Check sheet for the modelled part. Datum: model origin and axes. Units: mm. Face numbers are marked on the shaded views. Round coordinates to 2 decimals unless told otherwise and drop trailing zeros. Order: outer loops, then holes, each group sorted by start corner. A loop starts at its lowest first (then second) coordinate and runs counter-clockwise, first axis right, second up. Notation, with made-up numbers: (-5.5, 1.25) -> (37.5, 1.25) arc R15 ccw to (37.5, 17.25) -> close; hole circle Ø8 at (33, 4). An arc over 180 degrees is marked (long way). Answer in a Markdown table with one row per item. Add a question column.
1. Draft check along Y on the marked faces 1, 2 and 3. Enter one of: +Y half, -Y half, draft (parallel to the pull), parting line (faces both ways), or undercut.
2. Material ranges on L1, parallel to Z at x = 12.75, y = 20; L2, parallel to Z at x = 12.5, y = 15; L3, parallel to Y at x = 1.5, z = 34, recorded low to high. Write a range as from..to.
3. Depth check by flat-ended pin: P1, Ø16, axis at y = 19.56, z = -27.17, coming from the +X side; P2, Ø1, axis at y = 15.5, z = 112.5, coming from the +X side; P3, Ø5, axis at y = 16, z = 119, coming from the +X side; P4, Ø9.5, axis at y = 19.56, z = 137.83, coming from the -X side. Enter the tip coordinate at first touch or a pass-through.
4. Sectioned sample at B-B, the plane y = 17. Record the boundary of the cut face in (x, z).
5. Sectioned sample at A-A, the plane x = 1.75. Record the boundary of the cut face in (y, z), then the cut area to 3 significant figures.
6. Sectioned sample at D-D, the plane x = 12. Record the boundary of the cut face in (y, z).
7. Sectioned sample at C-C, the plane z = 106.5. Record the boundary of the cut face in (x, y).
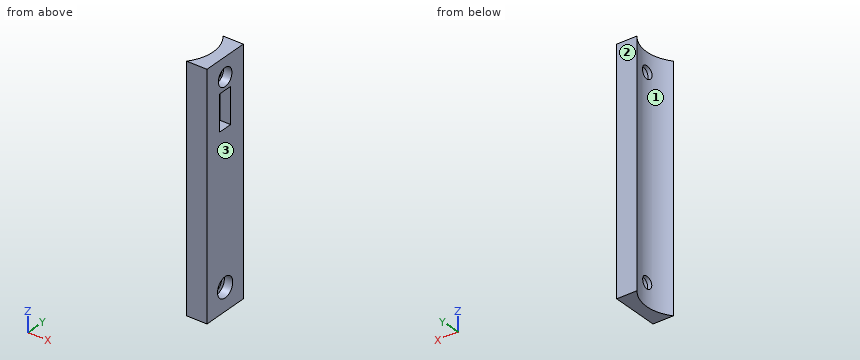
```python
from build123d import *
from build123d import SkipClean  # not in build123d's __all__

# Parameters (mm, degrees)
F0_W      = 40
F0_H      = 200
F1_DEPTH  = 17
F2_R      = 32
F3_DEPTH  = 187
F4_DEPTH  = 195
F5_R      = 8.3828490824
F5_R_2    = 7.5
F6_DEPTH  = 7
F7_R      = 5
F7_R_2    = 5.25
F8_DEPTH  = 25
F9_W      = 12
F9_H      = 30
F10_DEPTH = 9


with BuildPart() as f1:
    # F0 (on Right) → F1 (new body)
    with BuildSketch(Plane.YZ):
        with Locations((19.5646310411, 53.8327481339)):
            Rectangle(F0_W, F0_H)
    extrude(amount=F1_DEPTH)

    # F2 (on Top) → F3 (cut, symmetric)
    with BuildSketch(Plane.XY):
        with Locations((-24.9799919936, 19.5646310411)):
            Circle(F2_R)
    extrude(amount=F3_DEPTH, both=True, mode=Mode.SUBTRACT)

    # F2 (on Top) → F4 (cut)
    with BuildSketch(Plane.XY):
        with Locations((-24.9799919936, 19.5646310411)):
            Circle(F2_R)
    extrude(amount=-F4_DEPTH, mode=Mode.SUBTRACT)

    # F5 (on face) → F6 (cut)
    with BuildSketch(Plane.YZ.offset(17)):
        with Locations((19.5646310411, -27.1672518661)):
            Circle(F5_R)
        with Locations((19.5646310411, 137.8327481339)):
            Circle(F5_R_2)
    extrude(amount=-F6_DEPTH, mode=Mode.SUBTRACT)

    # F7 (on face) → F8 (cut)
    with BuildSketch(Plane.YZ.offset(10)):
        with Locations((19.5646310411, -27.1672518661)):
            Circle(F7_R)
        with Locations((19.5646310411, 137.8327481339)):
            Circle(F7_R_2)
    with SkipClean():  # cleaning this boolean's faces spoils the solid; the shape is the same uncleaned
        extrude(amount=-F8_DEPTH, mode=Mode.SUBTRACT)

    # F9 (on face) → F10 (cut)
    with BuildSketch(Plane.YZ.offset(17)):
        with Locations((19.5646310411, 112.5827481339)):
            Rectangle(F9_W, F9_H)
    with SkipClean():  # cleaning this boolean's faces spoils the solid; the shape is the same uncleaned
        extrude(amount=-F10_DEPTH, mode=Mode.SUBTRACT)


solid = f1.part
```
Answer key:
| question | item | result |
|---|---|---|
| 1 | face 1 | undercut |
| 1 | face 2 | +Y half |
| 1 | face 3 | draft |
| 2 | L1 | z = -46.17..-35.54, -18.8..97.58, 127.58..130.35, 145.32..153.83 |
| 2 | L2 | z = -46.17..-34.2, -20.14..97.58, 127.58..131.88, 143.78..153.83 |
| 2 | L3 | y = -0.44..1.6, 37.53..39.56 |
| 3 | P1 | stops at x = 10 |
| 3 | P2 | stops at x = 8 |
| 3 | P3 | stops at x = 17 |
| 3 | P4 | passes through |
| 4 | outline | (6.92, -46.17) -> (17, -46.17) -> (17, -35.15) -> (10, -35.15) -> (10, -31.46) -> (6.92, -31.46) -> close; (6.92, -22.88) -> (10, -22.88) -> (10, -19.19) -> (17, -19.19) -> (17, 97.58) -> (8, 97.58) -> (8, 127.58) -> (17, 127.58) -> (17, 130.78) -> (10, 130.78) -> (10, 133.25) -> (6.92, 133.25) -> close; (6.92, 142.41) -> (10, 142.41) -> (10, 144.88) -> (17, 144.88) -> (17, 153.83) -> (6.92, 153.83) -> close |
| 5 | outline | (-0.44, -46.17) -> (1.97, -46.17) -> (1.97, 153.83) -> (-0.44, 153.83) -> close; (37.16, -46.17) -> (39.56, -46.17) -> (39.56, 153.83) -> (37.16, 153.83) -> close |
| 5 | area | 963 mm² |
| 6 | outline | (-0.44, -46.17) -> (39.56, -46.17) -> (39.56, 153.83) -> (-0.44, 153.83) -> close; hole circle Ø16.77 at (19.56, -27.17); hole circle Ø15 at (19.56, 137.83); hole (13.56, 97.58) -> (25.56, 97.58) -> (25.56, 127.58) -> (13.56, 127.58) -> close |
| 7 | outline | (0, -0.44) -> (17, -0.44) -> (17, 13.56) -> (8, 13.56) -> (8, 25.56) -> (17, 25.56) -> (17, 39.56) -> (0, 39.56) arc R32 cw to start |
